```python
from build123d import *

# Parameters (mm, degrees)
BOSS_EXTRUDE4_DEPTH     = 15
SKETCH9_R               = 4
CUT_EXTRUDE2_DEPTH      = 151
CUT_EXTRUDE2_DEPTH_BACK = 151
BOSS_EXTRUDE6_START     = 150
SKETCH10_R              = 4
BOSS_EXTRUDE6_DEPTH     = 10
BOSS_EXTRUDE7_START     = -150
SKETCH12_R              = 4
BOSS_EXTRUDE7_DEPTH     = 10
SKETCH14_W              = 10
SKETCH14_H              = 50
BOSS_EXTRUDE8_DEPTH     = 50
SKETCH15_R              = 2
SKETCH15_R_2            = 12.5
CUT_EXTRUDE3_DEPTH      = 10


with BuildPart() as part:
    # Sketch8 → Boss-Extrude4 (new body)
    with BuildSketch(Plane(origin=(0, 0, 0), x_dir=(1, 0, 0), z_dir=(0, 1, 0))):
        with BuildLine():
            Line((-150, 50), (-150, 80))
            ThreePointArc((-150, 80), (-144.142135624, 94.142135624), (-130, 100))
            Line((-130, 100), (30, 100))
            ThreePointArc((30, 100), (44.142135624, 94.142135624), (50, 80))
            Line((50, 80), (50, 70))
            ThreePointArc((50, 70), (55.857864376, 55.857864376), (70, 50))
            Line((70, 50), (150, 50))
            Line((150, 50), (150, -50))
            Line((150, -50), (-150, -50))
            Line((-150, -50), (-150, 50))
        make_face()
    extrude(amount=BOSS_EXTRUDE4_DEPTH)

    # Sketch9 → Cut-Extrude2 (cut, two sides)
    with BuildSketch(Plane(origin=(0, 0, 0), x_dir=(0, 0, -1), z_dir=(1, 0, 0))) as cut_extrude2_sk:
        with Locations((-40, 7.5)):
            Circle(SKETCH9_R)
        with Locations((40, 7.5)):
            Circle(SKETCH9_R)
    extrude(amount=CUT_EXTRUDE2_DEPTH, mode=Mode.SUBTRACT)
    extrude(cut_extrude2_sk.sketch, amount=-CUT_EXTRUDE2_DEPTH_BACK, mode=Mode.SUBTRACT)

    # Sketch10 → Boss-Extrude6 (add)
    with BuildSketch(Plane(origin=(0, 0, 0), x_dir=(0, 0, -1), z_dir=(1, 0, 0)).offset(BOSS_EXTRUDE6_START)):
        with BuildLine():
            Line((-50, 15), (50, 15))
            Line((50, 15), (15.340491406, 153.638034376))
            ThreePointArc((15.340491406, 153.638034376), (10.019537045, 161.82308157), (0.788353904, 165))
            Line((0.788353904, 165), (-0.788353904, 165))
            ThreePointArc((-0.788353904, 165), (-10.019537045, 161.82308157), (-15.340491406, 153.638034376))
            Line((-15.340491406, 153.638034376), (-50, 15))
        make_face()
        with Locations((0, 150)):
            Circle(SKETCH10_R, mode=Mode.SUBTRACT)
        Polygon((-32.038353904, 25), (32.038353904, 25), (5.788353904, 130), (-5.788353904, 130), align=None, mode=Mode.SUBTRACT)
    extrude(amount=-BOSS_EXTRUDE6_DEPTH)

    # Sketch12 → Boss-Extrude7 (add)
    with BuildSketch(Plane(origin=(0, 0, 0), x_dir=(0, 0, -1), z_dir=(1, 0, 0)).offset(BOSS_EXTRUDE7_START)):
        with BuildLine():
            Line((-50, 15), (50, 15))
            Line((50, 15), (15.340491406, 153.638034376))
            ThreePointArc((15.340491406, 153.638034376), (10.019537045, 161.82308157), (0.788353904, 165))
            Line((0.788353904, 165), (-0.788353904, 165))
            ThreePointArc((-0.788353904, 165), (-10.019537045, 161.82308157), (-15.340491406, 153.638034376))
            Line((-15.340491406, 153.638034376), (-50, 15))
        make_face()
        with Locations((0, 150)):
            Circle(SKETCH12_R, mode=Mode.SUBTRACT)
        Polygon((-32.038353904, 25), (32.038353904, 25), (5.788353904, 130), (-5.788353904, 130), align=None, mode=Mode.SUBTRACT)
    extrude(amount=BOSS_EXTRUDE7_DEPTH)

    # Sketch14 → Boss-Extrude8 (add)
    with BuildSketch(Plane(origin=(0, 15, 0), x_dir=(1, 0, 0), z_dir=(0, 1, 0))):
        with Locations((-83, 75)):
            Rectangle(SKETCH14_W, SKETCH14_H)
    extrude(amount=BOSS_EXTRUDE8_DEPTH)

    # Sketch15 → Cut-Extrude3 (cut)
    with BuildSketch(Plane.ZY.offset(88)):
        with Locations((-90.5, 57.610296458)):
            Circle(SKETCH15_R)
        with Locations((-59.5, 57.610296458)):
            Circle(SKETCH15_R)
        with Locations((-90.5, 22.389703542)):
            Circle(SKETCH15_R)
        with Locations((-59.5, 22.389703542)):
            Circle(SKETCH15_R)
        with Locations((-74.409733022, 40)):
            Circle(SKETCH15_R_2)
    extrude(amount=-CUT_EXTRUDE3_DEPTH, mode=Mode.SUBTRACT)


solid = part.part
```
CAD build for the part. Positions are in the model's coordinates, mm. A direction names the side the tool comes from. Coordinates: 2 decimals unless noted, no trailing zeros. Loops run counter-clockwise (first coordinate to the right, second up) from the corner with the lowest first, then second, coordinate; pieces in that order, holes last. Notation, with made-up numbers: (17, 78) - (30, 78) arc R25 cw to (30, 104) - close; hole circle Ø5 at (5.25, 87). An arc over 180 degrees is marked (long way). Use CSV: the item, a comma, the result in double quotes. Start each with the question number.
Q1. Cut at B-B, the plane x = -124. List the corners of the cut face in (y, z).
Q2. 3-axis set-ups, long thin cutter, end or side, ignore diameter. For faces 4 (the flat face through (-145.07, 78.23, 18.73)), 5 (the flat face through (-78, 28.5, -80.2)), 6 (the flat face through (109, 7, -50)): which of +Z, -Z, +X, -X, +Y, -Y reach the whole face in a straight line?
Q3. Drop flat-ended pins along their axis: P1, Ø7.5, axis at x = 101.5, y = 7, coming from the -Z side; P2, Ø5, axis at x = -83.5, z = -68.5, coming from the +Y side; P3, Ø15, axis at y = 30, z = -68.5, coming from the +X side; P4, Ø22.5, axis at y = 40, z = -74.41, coming from the -X side. Give the stop position or say it passes through.
Q4. Cut at D-D, the plane z = 22.5. List the corners of the cut face in (x, y).
Q5. Cut at A-A, the plane y = 150. List the corners of the cut face in (x, z), then the cut area to 3 significant figures.
Q6. Two-plate mould, pull along Y, no slides. Class faces 1 (the cylindrical face through (43.986, 7.395, -94.297)), 2 (the cylindrical face through (-145.07, 161.737, -10.129)), 3 (the flat face through (145, 130, 0)): +Y half, -Y half, draft (parallel to the pull), parting line (faces both ways), or undercut.
Q7. Probe probe 1 along Y at (x, z) = (145, 0); probe 2 along Z at (x, y) = (-35.5, 7.5); probe 3 along Y at (x, z) = (-70, 40). List the from-to ranges inside material, lowest first. Write a range as from..to.
Q8. Cut at C-C, the plane y = 7.5. List the corners of the cut face in (x, z), then the cut area to 3 significant figures.
Here are the results:
1,outline,"(0, -100) - (15, -100) - (15, 50) - (0, 50) - close; hole circle Ø8 at (7.5, -40); hole circle Ø8 at (7.5, 40)"
2,face 4,"+X, -X"
2,face 5,"+Z, -Z, +X, +Y"
2,face 6,"-Z, +X, +Y, -Y"
3,P1,"z = -50"
3,P2,"y = 65"
3,P3,"x = -78"
3,P4,"through"
4,outline,"(-150, 0) - (150, 0) - (150, 25) - (140, 25) - (140, 15) - (-140, 15) - (-140, 25) - (-150, 25) - close; (-150, 63.15) - (-140, 63.15) - (-140, 125) - (-150, 125) - close; (140, 63.15) - (150, 63.15) - (150, 125) - (140, 125) - close"
5,outline,"(-150, -16.25) - (-140, -16.25) - (-140, -4) - (-150, -4) - close; (-150, 4) - (-140, 4) - (-140, 16.25) - (-150, 16.25) - close; (140, -16.25) - (150, -16.25) - (150, -4) - (140, -4) - close; (140, 4) - (150, 4) - (150, 16.25) - (140, 16.25) - close"
5,area,"490 mm2"
6,face 1,"draft"
6,face 2,"+Y half"
6,face 3,"undercut"
7,probe 1,"0..25, 130..146, 154..165"
7,probe 2,"-100..-44, -36..36, 44..50"
7,probe 3,"0..3.5, 11.5..15"
8,outline,"(-150, -80) arc R20 ccw to (-130, -100) - (30, -100) arc R20 ccw to (50, -80) - (50, -70) arc R20 cw to (70, -50) - (150, -50) - (150, -44) - (-150, -44) - close; (-150, -36) - (150, -36) - (150, 36) - (-150, 36) - close; (-150, 44) - (150, 44) - (150, 50) - (-150, 50) - close"
8,area,"35,100 mm2"
